```python
from build123d import *

# Parameters (mm, degrees)
F0_R            = 27.5
F0_R_2          = 5
F1_DEPTH        = 15
F2_R            = 2
F3_DEPTH        = 15.001
F3_COPIES_COUNT = 9


# Not quite as in the source:
# - a pattern or mirror of a feature is missing from the dataset's text; its kind, count and spacing are read off the source's solid


with BuildPart() as f1:
    # F0 (on Top) → F1 (new body)
    with BuildSketch(Plane.XY):
        Circle(F0_R)
        Circle(F0_R_2, mode=Mode.SUBTRACT)
    extrude(amount=F1_DEPTH)

    # F2 (on face) → F3 (cut, through all)
    with BuildSketch(Plane.XY.offset(15)):
        with Locations((15, 0)):
            Circle(F2_R)
    f3 = extrude(amount=-F3_DEPTH, mode=Mode.SUBTRACT)

    # F3_copies: F3 ×9 about axis
    f3_copies_axis = Axis((0, 0, 0), (0, 0, 1))
    for i in range(1, F3_COPIES_COUNT):
        add(f3.rotate(f3_copies_axis, i * 360 / F3_COPIES_COUNT), mode=Mode.SUBTRACT)


solid = f1.part
```
Work out the finished part from the listing and answer in its coordinate system (mm). Give positions to 0.01 mm unless a question says otherwise; leave off trailing zeros. Write each loop counter-clockwise with the first axis right and the second up, starting at its lowest first coordinate (ties: lowest second). Pieces come first, ordered by that corner, then holes.
(1) The part is cut by section A-A on y = 0. Write down the section's boundary in (x, z), plus the area to 3 significant figures.
Final values:
outline: (-27.5, 0) - (-5, 0) - (-5, 15) - (-27.5, 15) - close; (5, 0) - (13, 0) - (13, 15) - (5, 15) - close; (17, 0) - (27.5, 0) - (27.5, 15) - (17, 15) - close
area: 615 mm2
(2) The part is cut by section C-C on z = 7.75. Count the separate pieces of the cut face and the enclosed holes in it, plus the area to 3 significant figures.
Final values:
separate pieces: 1
enclosed holes: 10
area: 2,180 mm2
(3) The part is cut by section D-D on x = 2. Write down the section's boundary in (y, z).
Final values:
outline: (-27.43, 0) - (-16.68, 0) - (-16.68, 15) - (-27.43, 15) - close; (-12.87, 0) - (-4.58, 0) - (-4.58, 15) - (-12.87, 15) - close; (4.58, 0) - (12.87, 0) - (12.87, 15) - (4.58, 15) - close; (16.68, 0) - (27.43, 0) - (27.43, 15) - (16.68, 15) - close
(4) Straight lines are drawn through the part: line 1 (Y direction, x = -8, z = 13.25); line 2 (Y direction, x = 10.5, z = 13.25); line 3 (Y direction, x = 0, z = 7.25). For each, find the intervals that lie inside material, in ascending order.
Final values:
line 1: y = -26.31 to -14.93, -11.05 to 11.05, 14.93 to 26.31
line 2: y = -25.42 to -11.38, -7.9 to 7.9, 11.38 to 25.42
line 3: y = -27.5 to -5, 5 to 27.5
(5) The part is cut by section B-B on x = -7.5. Write down the section's boundary in (y, z), plus the area to 3 significant figures.
Final values:
outline: (-26.46, 0) - (-14.99, 0) - (-14.99, 15) - (-26.46, 15) - close; (-10.99, 0) - (10.99, 0) - (10.99, 15) - (-10.99, 15) - close; (14.99, 0) - (26.46, 0) - (26.46, 15) - (14.99, 15) - close
area: 674 mm2
(6) The mould has two halves that part along Y. Classify faces 1 (the cylindrical face through (-16.093, 5.218, 7.605)), 2 (the cylindrical face through (-5.961, -26.846, 7.395)), 3 (the cylindrical face through (2.344, 16.755, 7.605)), 4 (the flat face through (6, 0, 15)): pulls with the +Y half, pulls with the -Y half, needs draft (parallel to the pull), parting line crosses it, or undercut.
Final values:
face 1: undercut
face 2: parting line crosses it
face 3: undercut
face 4: needs draft
(7) Flat-ended cylindrical pins translate along their axes: pin 1 Ø3 at (y, z) = (-5.5, 7.5) entering from -X; pin 2 Ø8 at (y, z) = (-19.5, 3.5) entering from +X; pin 3 Ø1.5 at (y, z) = (-11.5, 6) entering from +X. Find the tip coordinate at first contact, or state that the pin passes through.
Final values:
pin 1: stops at x = -27.21
pin 2: stops at x = 22.72
pin 3: stops at x = 25.31
